```python
from build123d import *

# Parameters (mm, degrees)
SKETCH1_W                = 64
SKETCH1_H                = 42
BOSS_EXTRUDE1_DEPTH      = 7
SKETCH11_W               = 22
SKETCH11_H               = 16
BOSS_EXTRUDE3_DEPTH      = 7
BOSS_EXTRUDE3_DEPTH_BACK = 20
SKETCH3_R                = 12
CUT_EXTRUDE2_DEPTH       = 3
SKETCH2_R                = 4.1
CUT_EXTRUDE1_DEPTH       = 28
SKETCH4_R                = 2.75
CUT_EXTRUDE3_DEPTH       = 28
SKETCH7_R                = 1.65
CUT_EXTRUDE5_DEPTH       = 28
SKETCH8_W                = 42
SKETCH8_H                = 27
BOSS_EXTRUDE2_DEPTH      = 7
SKETCH9_R                = 2.7
CUT_EXTRUDE6_DEPTH       = 1
CUT_EXTRUDE6_DEPTH_BACK  = 13
SKETCH10_R               = 5
CUT_EXTRUDE7_DEPTH       = 20
SKETCH15_R               = 2.15
CUT_EXTRUDE8_DEPTH       = 22
SKETCH16_W               = 14
SKETCH16_H               = 3
CUT_EXTRUDE9_DEPTH       = 28
FILLET1_R                = 3
FILLET2_R                = 5


with BuildPart() as part:
    # Sketch1 → Boss-Extrude1 (new body)
    with BuildSketch(Plane(origin=(0, 0, 0), x_dir=(1, 0, 0), z_dir=(0, 1, 0))):
        Rectangle(SKETCH1_W, SKETCH1_H)
    extrude(amount=BOSS_EXTRUDE1_DEPTH)

    # Sketch11 → Boss-Extrude3 (add, two sides)
    with BuildSketch(Plane(origin=(0, 0, 0), x_dir=(1, 0, 0), z_dir=(0, 1, 0))) as boss_extrude3_sk:
        with Locations((43, 0)):
            Rectangle(SKETCH11_W, SKETCH11_H)
    extrude(amount=BOSS_EXTRUDE3_DEPTH)
    extrude(boss_extrude3_sk.sketch, amount=-BOSS_EXTRUDE3_DEPTH_BACK)

    # Sketch3 → Cut-Extrude2 (cut)
    with BuildSketch(Plane(origin=(0, 0, 0), x_dir=(1, 0, 0), z_dir=(0, 1, 0))):
        with Locations((10, 0)):
            Circle(SKETCH3_R)
    extrude(amount=CUT_EXTRUDE2_DEPTH, mode=Mode.SUBTRACT)

    # Sketch2 → Cut-Extrude1 (cut, through all)
    with BuildSketch(Plane(origin=(0, 7, 0), x_dir=(1, 0, 0), z_dir=(0, 1, 0))):
        with Locations((40, 0)):
            Circle(SKETCH2_R)
    extrude(amount=-CUT_EXTRUDE1_DEPTH, mode=Mode.SUBTRACT)

    # Sketch4 → Cut-Extrude3 (cut, through all)
    with BuildSketch(Plane(origin=(0, 7, 0), x_dir=(1, 0, 0), z_dir=(0, 1, 0))):
        with Locations((-22, 11)):
            Circle(SKETCH4_R)
        with Locations((-22, -11)):
            Circle(SKETCH4_R)
    extrude(amount=-CUT_EXTRUDE3_DEPTH, mode=Mode.SUBTRACT)

    # Sketch7 → Cut-Extrude5 (cut, through all)
    with BuildSketch(Plane(origin=(0, 7, 0), x_dir=(1, 0, 0), z_dir=(0, 1, 0))):
        with Locations((-5.5, 15.5)):
            Circle(SKETCH7_R)
        with Locations((25.5, 15.5)):
            Circle(SKETCH7_R)
        with Locations((25.5, -15.5)):
            Circle(SKETCH7_R)
        with Locations((-5.5, -15.5)):
            Circle(SKETCH7_R)
    extrude(amount=-CUT_EXTRUDE5_DEPTH, mode=Mode.SUBTRACT)

    # Sketch8 → Boss-Extrude2 (add)
    with BuildSketch(Plane.ZY.offset(32)):
        with Locations((0, -6.5)):
            Rectangle(SKETCH8_W, SKETCH8_H)
    extrude(amount=BOSS_EXTRUDE2_DEPTH)

    # Sketch9 → Cut-Extrude6 (cut, two sides)
    with BuildSketch(Plane.ZY.offset(39)) as cut_extrude6_sk:
        with Locations((0, -10)):
            Circle(SKETCH9_R)
    extrude(amount=CUT_EXTRUDE6_DEPTH, mode=Mode.SUBTRACT)
    extrude(cut_extrude6_sk.sketch, amount=-CUT_EXTRUDE6_DEPTH_BACK, mode=Mode.SUBTRACT)

    # Sketch10 → Cut-Extrude7 (cut)
    with BuildSketch(Plane(origin=(0, 7, 0), x_dir=(1, 0, 0), z_dir=(0, 1, 0))):
        with Locations((10, 0)):
            Circle(SKETCH10_R)
    extrude(amount=-CUT_EXTRUDE7_DEPTH, mode=Mode.SUBTRACT)

    # Sketch15 → Cut-Extrude8 (cut)
    with BuildSketch(Plane(origin=(0, 0, -8), x_dir=(-1, 0, 0), z_dir=(0, 0, -1))):
        with Locations((-49, 0)):
            Circle(SKETCH15_R)
        with Locations((-49, -14)):
            Circle(SKETCH15_R)
    extrude(amount=-CUT_EXTRUDE8_DEPTH, mode=Mode.SUBTRACT)

    # Sketch16 → Cut-Extrude9 (cut, through all)
    with BuildSketch(Plane(origin=(0, 7, 0), x_dir=(1, 0, 0), z_dir=(0, 1, 0))):
        with Locations((47, 0)):
            Rectangle(SKETCH16_W, SKETCH16_H)
    extrude(amount=-CUT_EXTRUDE9_DEPTH, mode=Mode.SUBTRACT)

    # Fillet1
    fillet1_edges = [part.edges().sort_by_distance(p)[0] for p in [
        (32, 3.5, -8),
        (32, 3.5, 8),
    ]]
    fillet(fillet1_edges, radius=FILLET1_R)

    # Fillet2
    fillet2_edges = [part.edges().sort_by_distance(p)[0] for p in [
        (32, 3.5, 21),
        (32, 3.5, -21),
    ]]
    fillet(fillet2_edges, radius=FILLET2_R)


solid = part.part
```
Read the model definition and answer for the solid it produces. Units are mm, in the model's axes. A direction names the side the tool comes from. Give positions to 0.01 mm unless a question says otherwise; leave off trailing zeros. Write each loop counter-clockwise with the first axis right and the second up, starting at its lowest first coordinate (ties: lowest second). Pieces come first, ordered by that corner, then holes. Notation, with made-up numbers: (-20.75, 0) - (-16.75, 0) arc R27 ccw to (-16.75, 24) - close; hole circle Ø7 at (79, 20.5). An arc over 180 degrees is marked (long way). Write item = value, one per line. Start each with the question number.
Item 1: Find the intervals of material crossed by probe 1 along Y at (x, z) = (49, -4); probe 2 along X at (y, z) = (2, 15.5); probe 3 along Z at (x, y) = (43.5, 4), in increasing order. Write a range as [from, to].
Item 2: The mould has two halves that part along Y. Classify faces 1 (the flat face through (-2, 7, 0)), 2 (the cylindrical face through (-35.549, -12.395, 1.246)), 3 (the flat face through (-32, -5, 0)): +Y half, -Y half, draft (parallel to the pull), parting line (faces both ways), or undercut.
Item 3: Find section C-C (y = -17.5). Give the vertices of the cut face in (x, z), then the cut area to 3 significant figures.
Item 4: Find section A-A (x = 49). Give the vertices of the cut face in (y, z).
Item 5: Find section D-D (x = 10). Give the vertices of the cut face in (y, z), then the cut area to 3 significant figures.
Item 6: Find section B-B (x = -5.5). Give the vertices of the cut face in (y, z).
Item 7: A tool of negligible diameter and unlimited length cuts with its end or side. For faces 4 (the flat face through (32, 3, 14)), 5 (the flat face through (49, -6, -1.5)), 6 (the flat face through (9.8, 3, 5.2)), from which of +Z, -Z, +X, -X, +Y, -Y can it reach the whole face along a straight path? Write none if from no direction.
Item 8: Each of these flat-tipped pins is pushed along its axis until it touches: P1, Ø7, axis at x = 7, z = -3, coming from the -Y side; P2, Ø2.5, axis at y = 2, z = 14.5, coming from the +X side; P3, Ø5, axis at x = -22, z = 11, coming from the -Y side; P4, Ø11, axis at x = 38, y = -5, coming from the -Z side. Where does it stop, or does it pass through?
Response:
q1.probe_1 = [-20, -16.15], [-11.85, -2.15], [2.15, 7]
q1.probe_2 = [-39, -7.15], [-3.85, 23.85], [27.15, 32]
q1.probe_3 = [-8, -2.14], [2.14, 8]
q2.face_1 = +Y half
q2.face_2 = undercut
q2.face_3 = draft
q3.outline = (-39, -21) - (-32, -21) - (-32, 21) - (-39, 21) - close; (32, -8) - (54, -8) - (54, -1.5) - (43.82, -1.5) arc R4.1 cw (long way) to (43.82, 1.5) - (54, 1.5) - (54, 8) - (32, 8) - close
q3.area = 563 mm²
q4.outline = (-20, -8) - (-16.15, -8) - (-16.15, -1.5) - (-20, -1.5) - close; (-20, 1.5) - (-16.15, 1.5) - (-16.15, 8) - (-20, 8) - close; (-11.85, -8) - (-2.15, -8) - (-2.15, -1.5) - (-11.85, -1.5) - close; (-11.85, 1.5) - (-2.15, 1.5) - (-2.15, 8) - (-11.85, 8) - close; (2.15, -8) - (7, -8) - (7, -1.5) - (2.15, -1.5) - close; (2.15, 1.5) - (7, 1.5) - (7, 8) - (2.15, 8) - close
q5.outline = (0, -21) - (7, -21) - (7, -5) - (3, -5) - (3, -12) - (0, -12) - close; (0, 12) - (3, 12) - (3, 5) - (7, 5) - (7, 21) - (0, 21) - close
q5.area = 182 mm²
q6.outline = (0, -21) - (7, -21) - (7, -17.15) - (0, -17.15) - close; (0, -13.85) - (7, -13.85) - (7, 13.85) - (0, 13.85) - close; (0, 17.15) - (7, 17.15) - (7, 21) - (0, 21) - close
q7.face_4 = +Z, +X, +Y, -Y
q7.face_5 = +X, +Y, -Y
q7.face_6 = -Y
q8.P1 = 3
q8.P2 = 32
q8.P3 = through
q8.P4 = -8
